For this review, use the dimensioned drawing (mm, ordinates from the lowest corner) and the shaded views. A direction names the side the tool comes from. Give positions to 0.01 mm unless a question says otherwise; leave off trailing zeros. Order: outer loops, then holes, each group sorted by start corner. A loop starts at its lowest first (then second) coordinate and runs counter-clockwise, first axis right, second up.
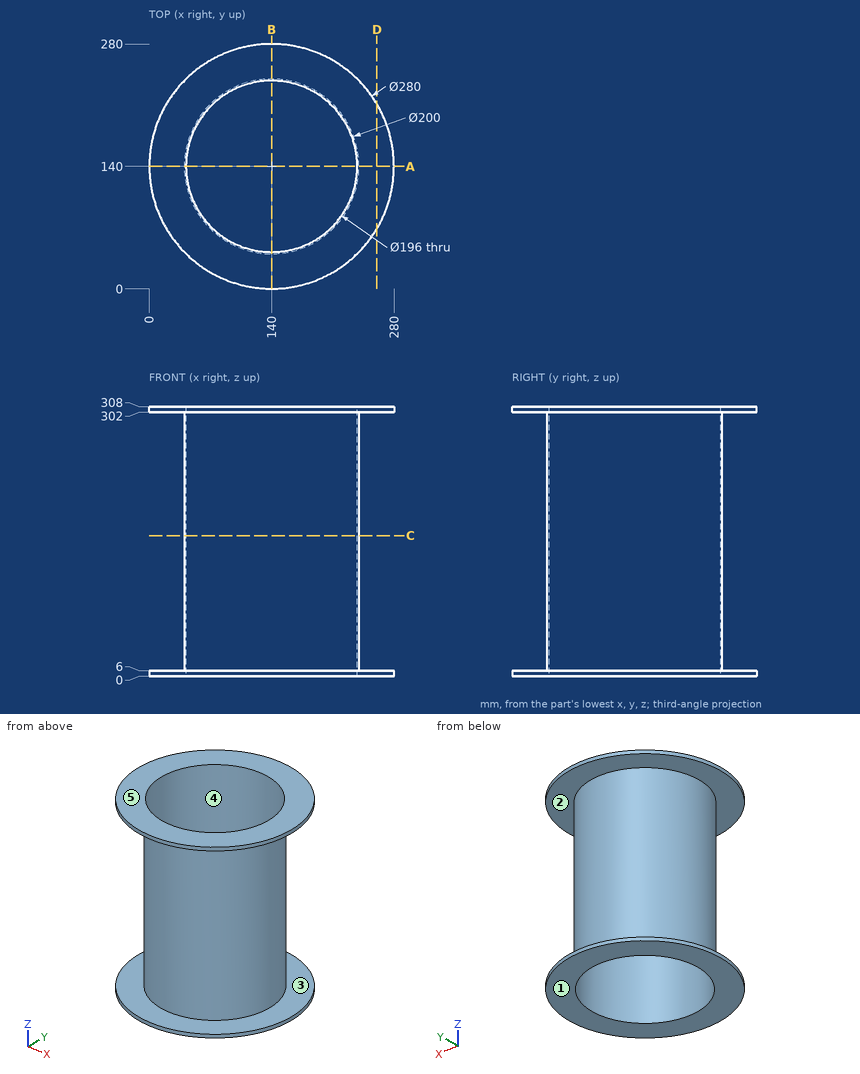
1. For line 1 along X through (y, z) = (142, 78); line 2 along Y through (x, z) = (140, 224.5); line 3 along Z through (x, y) = (45.5, 218.5), list the stretches that pass through material, from the lowest coordinate up.
Recorded:
line 1: x = 40.02 to 42.02, 237.98 to 239.98
line 2: y = 40 to 42, 238 to 240
line 3: z = 0 to 6, 302 to 308
2. For pin 1 (8 mm diameter, centred on x = 51.5, z = 82, fed in from +Y); pin 2 (4 mm diameter, centred on y = 218.5, z = 203, fed in from +X); pin 3 (4 mm diameter, centred on x = 120, z = 58, fed in from -Y), all flat-tipped, find the tip position at first contact; note any pin that passes through.
Recorded:
pin 1: stops at y = 193.48
pin 2: stops at x = 204.4
pin 3: stops at y = 41.63
3. Take a section at D-D (x = 260.5). State the section outline as (y, z) points, then the cut area to 3 significant figures.
Recorded:
outline: (68.73, 0) - (211.27, 0) - (211.27, 6) - (68.73, 6) - close; (68.73, 302) - (211.27, 302) - (211.27, 308) - (68.73, 308) - close
area: 1,710 mm2
4. Take a section at A-A (y = 140). State the section outline as (x, z) points.
Recorded:
outline: (0, 0) - (42, 0) - (42, 308) - (0, 308) - (0, 302) - (40, 302) - (40, 6) - (0, 6) - close; (238, 0) - (280, 0) - (280, 6) - (240, 6) - (240, 302) - (280, 302) - (280, 308) - (238, 308) - close
5. Take a section at C-C (z = 160.5). State the section outline as (x, y) points, then the cut area to 3 significant figures.
Recorded:
outline: circle Ø200 at (140, 140); hole circle Ø196 at (140, 140)
area: 1,240 mm2
6. Machinability: for the marked faces 1 and 2, which of the approach directions +Z, -Z, +X, -X, +Y, -Y give a long, thin tool a straight path to every point of the face, cutting with its end or side? Answer none if there is none.
Recorded:
face 1: -Z, +X, -X, +Y, -Y
face 2: none
7. Draft analysis for pull direction Z (two halves, no side actions). For the marked faces 3, 4 and 5, state which applies: pulls with the +Z half, pulls with the -Z half, needs draft (parallel to the pull), parting line crosses it, or undercut.
Recorded:
face 3: undercut
face 4: needs draft
face 5: pulls with the +Z half
